from build123d import *

# Parameters (mm, degrees)
SKETCH2_R           = 60
SKETCH2_R_2         = 35
BOSS_EXTRUDE1_DEPTH = 15
SKETCH3_R           = 51
CUT_EXTRUDE1_DEPTH  = 3
SKETCH4_W           = 6
SKETCH4_H           = 20
CUT_EXTRUDE2_DEPTH  = 10
CIRPATTERN1_COUNT   = 16
CHAMFER1_SIZE       = 4
SKETCH5_R           = 2
CUT_EXTRUDE3_DEPTH  = 86.697141143
SKETCH6_R           = 35
SKETCH6_R_2         = 1.75
SKETCH6_R_3         = 25
BOSS_EXTRUDE2_DEPTH = 2


with BuildPart() as part:
    # Sketch2 → Boss-Extrude1 (new body)
    with BuildSketch(Plane.XY):
        Circle(SKETCH2_R)
        Circle(SKETCH2_R_2, mode=Mode.SUBTRACT)
    extrude(amount=BOSS_EXTRUDE1_DEPTH)

    # Sketch3 → Cut-Extrude1 (cut)
    with BuildSketch(Plane.XY.offset(15)):
        Circle(SKETCH3_R)
    extrude(amount=-CUT_EXTRUDE1_DEPTH, mode=Mode.SUBTRACT)

    # Sketch4 → Cut-Extrude2 (cut)
    with BuildSketch(Plane.XY.offset(12)):
        with Locations((0, 51)):
            Rectangle(SKETCH4_W, SKETCH4_H)
    cut_extrude2 = extrude(amount=-CUT_EXTRUDE2_DEPTH, mode=Mode.SUBTRACT)

    # CirPattern1: Cut-Extrude2 ×16 about axis
    cirpattern1_axis = Axis((0, 0, 0), (0, 0, 1))
    for i in range(1, CIRPATTERN1_COUNT):
        add(cut_extrude2.rotate(cirpattern1_axis, i * 360 / CIRPATTERN1_COUNT), mode=Mode.SUBTRACT)

    # Chamfer1
    # the kernel refuses this chamfer: 4 mm, written as the material it takes off along each edge
    with BuildSketch(Plane(origin=(0, 0, 15), x_dir=(1, 0, 0), z_dir=(0, -1, 0))) as chamfer1_piece_1:
        Polygon((60, -CHAMFER1_SIZE), (60 - CHAMFER1_SIZE, 0), (60, 0), align=None)
    revolve(axis=Axis((0, 0, 15), (0, 0, 1)), mode=Mode.SUBTRACT)

    # Sketch5 → Cut-Extrude3 (cut, through all)
    with BuildSketch(Plane.XY.offset(12)):
        with Locations((25, -36)):
            Circle(SKETCH5_R)
        with Locations((-23, -36)):
            Circle(SKETCH5_R)
        with Locations((35, 24)):
            Circle(SKETCH5_R)
        with Locations((-35, 23)):
            Circle(SKETCH5_R)
    extrude(amount=-CUT_EXTRUDE3_DEPTH, mode=Mode.SUBTRACT)

    # Sketch6 → Boss-Extrude2 (add)
    with BuildSketch(Plane.XY):
        Circle(SKETCH6_R)
        with Locations((-30, 0)):
            Circle(SKETCH6_R_2, mode=Mode.SUBTRACT)
        Circle(SKETCH6_R_3, mode=Mode.SUBTRACT)
        with Locations((-27.716385975, 11.480502971)):
            Circle(SKETCH6_R_2, mode=Mode.SUBTRACT)
        with Locations((-21.213203436, 21.213203436)):
            Circle(SKETCH6_R_2, mode=Mode.SUBTRACT)
        with Locations((-11.480502971, 27.716385975)):
            Circle(SKETCH6_R_2, mode=Mode.SUBTRACT)
        with Locations((0, 30)):
            Circle(SKETCH6_R_2, mode=Mode.SUBTRACT)
        with Locations((11.480502971, 27.716385975)):
            Circle(SKETCH6_R_2, mode=Mode.SUBTRACT)
        with Locations((21.213203436, 21.213203436)):
            Circle(SKETCH6_R_2, mode=Mode.SUBTRACT)
        with Locations((27.716385975, 11.480502971)):
            Circle(SKETCH6_R_2, mode=Mode.SUBTRACT)
        with Locations((30, 0)):
            Circle(SKETCH6_R_2, mode=Mode.SUBTRACT)
        with Locations((27.716385975, -11.480502971)):
            Circle(SKETCH6_R_2, mode=Mode.SUBTRACT)
        with Locations((21.213203436, -21.213203436)):
            Circle(SKETCH6_R_2, mode=Mode.SUBTRACT)
        with Locations((11.480502971, -27.716385975)):
            Circle(SKETCH6_R_2, mode=Mode.SUBTRACT)
        with Locations((0, -30)):
            Circle(SKETCH6_R_2, mode=Mode.SUBTRACT)
        with Locations((-11.480502971, -27.716385975)):
            Circle(SKETCH6_R_2, mode=Mode.SUBTRACT)
        with Locations((-21.213203436, -21.213203436)):
            Circle(SKETCH6_R_2, mode=Mode.SUBTRACT)
        with Locations((-27.716385975, -11.480502971)):
            Circle(SKETCH6_R_2, mode=Mode.SUBTRACT)
    extrude(amount=BOSS_EXTRUDE2_DEPTH)


solid = part.part
Input: part model. Units: mm. Frame: model coordinates. A direction names the side the tool comes from. Coordinates: 2 decimals unless noted, no trailing zeros.
(1) Material intervals for probe 1 along Y at (x, z) = (-14.5, 2.25); probe 2 along Y at (x, z) = (32, 3.25); probe 3 along X at (y, z) = (-52.5, 7.5), sorted ascending.
(2) Set-up query: faces 1 (the face through (3, 50, 7)), 2 (the face through (11, -34, 12)), 3 (the face through (36, 36, 2)). Return all of +Z, -Z, +X, -X, +Y, -Y with unobstructed straight access to the full face (end or side cutting, diameter ignored); none if empty.
(3) Section A-A on y = 0. Count the separate pieces of the cut face and the enclosed holes in it, then the cut area to 3 significant figures.
(4) First-contact query: pin 1 Ø2 at (x, y) = (-9.5, -39.5) entering from +Z; pin 2 Ø8 at (x, z) = (1, 9) entering from -Y; pin 3 Ø5 at (y, z) = (15.5, 7) entering from -X. Flat tips, straight axial feed; report the tip coordinate or a pass-through.
Data:
1. probe 1: y = -58.22 to -42.85, -38.37 to -31.86, 31.86 to 38.37, 42.85 to 58.22
1. probe 2: y = -50.75 to -36.24, -27.76 to -14.18, 14.18 to 27.76, 36.24 to 50.75
1. probe 3: x = -29.05 to -24.99, -18.5 to -3, 3 to 18.5, 24.99 to 29.05
2. face 1: +Y
2. face 2: +Z
2. face 3: none
3. separate pieces: 6
3. enclosed holes: 0
3. area: 285 mm2
4. pin 1: stops at z = 12
4. pin 2: stops at y = -59.92
4. pin 3: stops at x = -58.57
